Geometry: see drawing. Coordinates: mm, zero at the bounding-box minimum. Round coordinates to 2 decimals unless told otherwise and drop trailing zeros. Write each loop counter-clockwise with the first axis right and the second up, starting at its lowest first coordinate (ties: lowest second). Pieces come first, ordered by that corner, then holes. Notation, with made-up numbers: (69, 22.25) -> (102, 22.25) arc R21 cw to (102, 54.25) -> close; hole circle Ø7 at (27, 75.5). An arc over 180 degrees is marked (long way). Use CSV: the item, a comma, the result in double quotes.
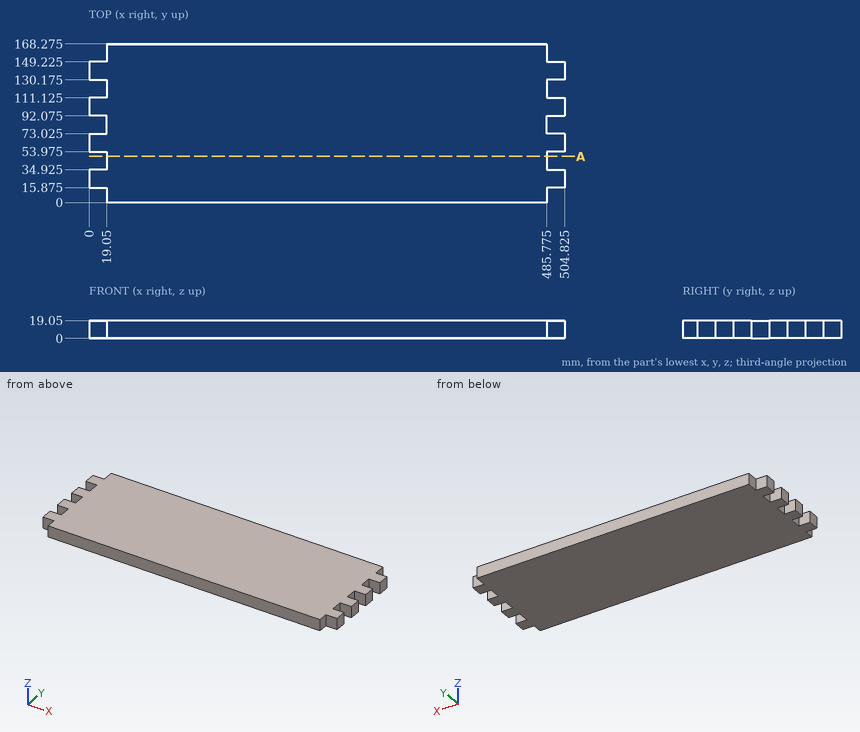
Item 1: First-contact query: pin 1 Ø5.5 at (y, z) = (46.5, 8.5) entering from -X; pin 2 Ø1 at (y, z) = (26.5, 7) entering from -X; pin 3 Ø1 at (y, z) = (38.5, 8) entering from +X (3 decimals); pin 4 Ø9.5 at (x, z) = (9.5, 6) entering from +Y (3 decimals). Flat tips, straight axial feed; report the tip coordinate or a pass-through.
Worked answers:
pin 1,"stops at x = 19.05"
pin 2,"stops at x = 0"
pin 3,"stops at x = 485.775"
pin 4,"stops at y = 149.225"
Item 2: Section query A-A on y = 49. Return the cut outline in (x, z) (3 decimals), plus the area to 3 significant figures.
Worked answers:
outline,"(19.05, 0) -> (485.775, 0) -> (485.775, 19.05) -> (19.05, 19.05) -> close"
area,"8,890 mm²"
Item 3: Line query: line 1 (X direction, y = 10.5, z = 9) (3 decimals). Output: solid intervals per line, ascending.
Worked answers:
line 1,"x = 19.05 to 485.775"
